```python
from build123d import *

# Parameters (mm, degrees)
BOSS_EXTRUDE1_DEPTH = 48
SKETCH2_W           = 12
SKETCH2_H           = 30
CUT_EXTRUDE1_DEPTH  = 18


with BuildPart() as part:
    # Sketch1 → Boss-Extrude1 (new body)
    with BuildSketch(Plane(origin=(0, 0, 0), x_dir=(1, 0, 0), z_dir=(0, 1, 0))):
        with BuildLine():
            Line((-44, 0), (-24, 0))
            Line((-24, 0), (-24, 12))
            Line((-24, 12), (-18.601840861, 12))
            ThreePointArc((-18.601840861, 12), (0, 30.601840861), (18.601840861, 12))
            Line((18.601840861, 12), (24, 12))
            Line((24, 12), (24, 0))
            Line((24, 0), (44, 0))
            Line((44, 0), (44, 12))
            Line((44, 12), (30, 40))
            Line((30, 40), (30, 58))
            Line((30, 58), (-30, 58))
            Line((-30, 58), (-30, 40))
            Line((-30, 40), (-44, 12))
            Line((-44, 12), (-44, 0))
        make_face()
    extrude(amount=-BOSS_EXTRUDE1_DEPTH)

    # Sketch2 → Cut-Extrude1 (cut)
    with BuildSketch(Plane(origin=(0, 0, -58), x_dir=(-1, 0, 0), z_dir=(0, 0, -1))):
        with Locations((-24, -23.945628859)):
            Rectangle(SKETCH2_W, SKETCH2_H)
    cut_extrude1 = extrude(amount=-CUT_EXTRUDE1_DEPTH, mode=Mode.SUBTRACT)

    # Mirror1: Cut-Extrude1 across plane
    add(cut_extrude1.mirror(Plane(origin=(0, 0, 0), x_dir=(0, 0, 1), z_dir=(1, 0, 0))), mode=Mode.SUBTRACT)


solid = part.part
```
Read the model definition and answer for the solid it produces. Units are mm, in the model's axes. A direction names the side the tool comes from. Give positions to 0.01 mm unless a question says otherwise; leave off trailing zeros. Order: outer loops, then holes, each group sorted by start corner. A loop starts at its lowest first (then second) coordinate and runs counter-clockwise, first axis right, second up.
(1) For faces 4 (the flat face through (30, -43, -49)), 5 (the flat face through (-24, -24, -6)), 6 (the flat face through (18, -24, -49)), determine the directions among +Z, -Z, +X, -X, +Y, -Y from which every point of the face is accessible in a straight line to the end or side of a thin tool.
(2) Given pin 1 (20 mm diameter, centred on y = -19, z = -49.5, fed in from +X); pin 2 (4.5 mm diameter, centred on y = -42.5, z = -50.5, fed in from -X); pin 3 (6 mm diameter, centred on x = 21.5, y = -12.5, fed in from +Z); pin 4 (4.5 mm diameter, centred on y = -41.5, z = -50.5, fed in from +X), each flat-ended and moving along its own axis, determine where each tip first touches the part or whether it passes through.
(3) Find section B-B (z = -25). Give the vertices of the cut face in (x, y), plus the area to 3 significant figures.
(4) Find section A-A (y = -21). Give the vertices of the cut face in (x, z).
(5) Find section C-C (z = -37.5). Give the vertices of the cut face in (x, y), plus the area to 3 significant figures.
(6) For a pull along X with two mould halves and no side action, classify faces 1 (the flat face through (-44, -24, -6)), 2 (the flat face through (34, -24, 0)), 3 (the flat face through (-21, -24, -12)) as released by +X, released by -X, zero draft, split by the parting line, or undercut.
(7) Find section D-D (x = 12). Give the vertices of the cut face in (y, z), plus the area to 3 significant figures.
(8) Straight lines are drawn through the part: L1, parallel to X at y = -28, z = -9.5; L2, parallel to Y at x = -27, z = -53; L3, parallel to Z at x = 25.5, y = -31.5. For each, find the intervals that lie inside material, in ascending order.
Result sheet:
1. face 4: -Z, +X, +Y, -Y
1. face 5: +Z, +Y, -Y
1. face 6: -Z, +X
2. pin 1: stops at x = 30.25
2. pin 2: stops at x = -30
2. pin 3: stops at z = 0
2. pin 4: stops at x = 30
3. outline: (-37.5, -48) - (-13.31, -48) - (-13.31, 0) - (-37.5, 0) - close; (13.31, -48) - (37.5, -48) - (37.5, 0) - (13.31, 0) - close
3. area: 2,320 mm2
4. outline: (-44, -12) - (-30, -40) - (-18, -40) - (-18, -58) - (18, -58) - (18, -40) - (30, -40) - (44, -12) - (44, 0) - (24, 0) - (24, -12) - (18.6, -12) arc R18.6 cw to (-18.6, -12) - (-24, -12) - (-24, 0) - (-44, 0) - close
5. outline: (-31.25, -48) - (31.25, -48) - (31.25, 0) - (-31.25, 0) - close
5. area: 3,000 mm2
6. face 1: released by -X
6. face 2: zero draft
6. face 3: undercut
7. outline: (-48, -58) - (0, -58) - (0, -26.21) - (-48, -26.21) - close
7. area: 1,530 mm2
8. L1: x = -44 to -24, 24 to 44
8. L2: y = -48 to -38.95, -8.95 to 0
8. L3: z = -40 to 0
